Study the drawing (mm; zero at the part's minimum x, y, z) and answer. Give positions to 0.01 mm unless a question says otherwise; leave off trailing zeros. Order: outer loops, then holes, each group sorted by start corner. A loop starts at its lowest first (then second) coordinate and runs counter-clockwise, first axis right, second up. Notation, with made-up numbers: (61.5, 28) - (88.5, 28) arc R26 cw to (88.5, 66) - close; hole circle Ø1 at (6.5, -33). An arc over 180 degrees is marked (long way). Return JSON: item names as keys, results as strings.
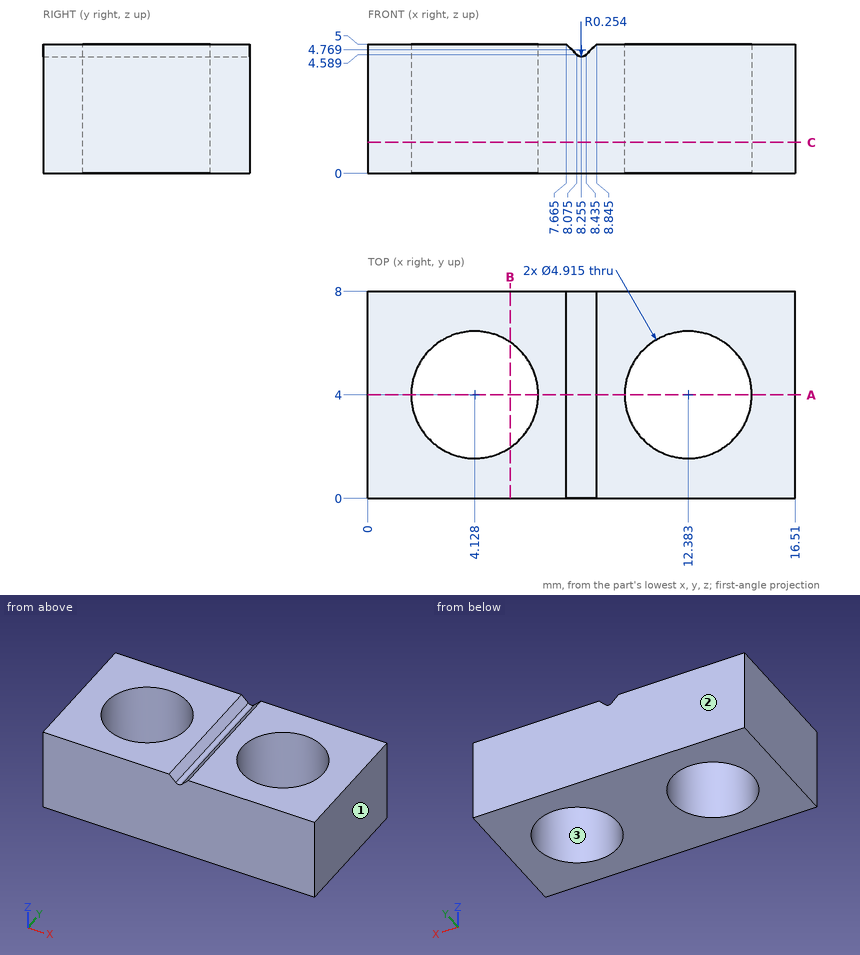
Q1. A cutting plane is placed at C-C (z = 1.2). Write down the section's boundary in (x, y) (1 decimal).
Values:
{"outline": "(0, 0) - (16.5, 0) - (16.5, 8) - (0, 8) - close; hole circle Ø4.9 at (4.1, 4); hole circle Ø4.9 at (12.4, 4)"}
Q2. A cutting plane is placed at A-A (y = 4). Give the number of separate pieces and of enclosed holes in the cut face.
Values:
{"separate pieces": "3", "enclosed holes": "0"}
Q3. Determine the mould class of the marked faces 1, 2 and 3 for opening direction Y: released by +Y, released by -Y, zero draft, split by the parting line, or undercut.
Values:
{"face 1": "zero draft", "face 2": "released by +Y", "face 3": "undercut"}
Q4. Given pin 1 (2 mm diameter, centred on y = 6, z = 0.5, fed in from -X); pin 2 (4 mm diameter, centred on x = 4.13, y = 4, fed in from -Z), each flat-ended and moving along its own axis, determine where each tip first touches the part or whether it passes through.
Values:
{"pin 1": "stops at x = 0", "pin 2": "passes through"}
Q5. A cutting plane is placed at B-B (x = 5.5). Write down the section's boundary in (y, z), and give its area (3 significant figures).
Values:
{"outline": "(0, 0) - (1.96, 0) - (1.96, 5) - (0, 5) - close; (6.04, 0) - (8, 0) - (8, 5) - (6.04, 5) - close", "area": "19.6 mm²"}
Q6. Consider L1, parallel to X at y = 3, z = 4.6 (1 decimal); L2, parallel to X at y = 6.25, z = 1 (1 decimal); L3, parallel to X at y = 2, z = 3.4 (1 decimal). Determine where each line is inside the solid, lowest interval first.
Values:
{"L1": "x = 0 to 1.9, 6.4 to 8.1, 8.4 to 10.1, 14.6 to 16.5", "L2": "x = 0 to 3.1, 5.1 to 11.4, 13.4 to 16.5", "L3": "x = 0 to 2.7, 5.6 to 11, 13.8 to 16.5"}
